Read the model definition and answer for the solid it produces. Units are mm, in the model's axes. Face numbers are marked on the shaded views. A direction names the side the tool comes from. Coordinates: 2 decimals unless noted, no trailing zeros. Loops run counter-clockwise (first coordinate to the right, second up) from the corner with the lowest first, then second, coordinate; pieces in that order, holes last. Notation, with made-up numbers: (76.25, 15.25) - (87.25, 15.25) arc R24 ccw to (87.25, 28.25) - close; hole circle Ø7 at (78.25, 40). An arc over 180 degrees is marked (long way). Use CSV: the item, a comma, the result in double quotes.
Autodesk Inventor part; units mm, degrees
ref_plane "YZ Plane" through (0, 0, 0) normal (1, 0, 0) x (0, 1, 0)
ref_plane "XZ Plane" through (0, 0, 0) normal (0, 1, 0) x (-1, 0, 0)
ref_plane "XY Plane" through (0, 0, 0) normal (0, 0, 1) x (1, 0, 0)
sketch "Skizze7" plane through (0, 0, 0) normal (0, -1, 0) x (1, 0, 0)
  point P0 (-1.8443, 26.478)
sketch "Skizze1" plane through (0, 0, 0) normal (0, 1, 0) x (-1, 0, 0)
  arc A0 (-2.1739, -19.8815) -> (-2.1739, 19.8815) centre (0, 0) ccw
  arc A1 (-47.6304, 14.9111) -> (-47.6304, -14.9111) centre (-46, 0) ccw
  line L0 (-2.1739, 19.8815) -> (-47.6304, 14.9111)
  line L1 (-2.1739, -19.8815) -> (-47.6304, -14.9111)
  line L2 (45.0235, 0) -> (-115.148, 0) construction
  dimension "d0" = 40
  dimension "d1" = 30
  dimension "d2" = 46
extrude "Extrusion1" add sketch "Skizze1" along normal blind 5
shell "Wandung1" thickness 3 removed faces 1 at (17.3261, 5, -4.9704)
sketch "Skizze2" plane through (0, 3, 0) normal (0, 1, 0) x (1, 0, 0)
  circle A0 centre (0, 0) radius 9.5
  circle A1 centre (0, 0) radius 12
  dimension "d6" = 19
  dimension "d7" = 24
extrude "Extrusion2" add sketch "Skizze2" along normal blind 3
sketch "Skizze3" plane through (0, 3, 0) normal (0, 1, 0) x (1, 0, 0)
  arc A0 (47.3043, -11.9289) -> (47.3043, 11.9289) centre (46, 0) ccw
  circle A1 centre (46, 0) radius 9.5
  circle A2 centre (46, 0) radius 12
  point P0 (0, 0)
  point P1 (47.3043, -11.9289)
  dimension "d10" = 19
extrude "Extrusion3" add sketch "Skizze3" along normal blind 3
sketch "Skizze4" plane through (0, 3, 0) normal (0, 1, 0) x (1, 0, 0)
  circle A0 centre (0, 0) radius 9.5
extrude "Extrusion4" cut sketch "Skizze4" against normal blind 2
sketch "Skizze5" plane through (46, 3, 0) normal (0, 1, 0) x (1, 0, 0)
  circle A0 centre (0, 0) radius 9.5
  point P0 (-46, 0)
extrude "Extrusion5" cut sketch "Skizze5" against normal blind 2
sketch "Skizze6" plane through (46, 1, 0) normal (0, 1, 0) x (1, 0, 0)
  point P0 (-46, 0)
  point P1 (0, 0)
  point P2 (0, 0)
hole "Bohrung1" at (46, 1, 0) direction (0, -1, 0) diameter 11 end through all
sketch "Skizze8" plane through (0, 5, 0) normal (0, 1, 0) x (1, 0, 0)
  arc A0 (1.8478, 16.8993) -> (1.8478, -16.8993) centre (0, 0) ccw
  arc A1 (2.1739, 19.8815) -> (2.1739, -19.8815) centre (0, 0) ccw
  line L0 (47.3043, -11.9289) -> (1.8478, -16.8993)
  line L1 (2.1739, -19.8815) -> (47.6304, -14.9111)
  arc A2 (47.6304, -14.9111) -> (47.6304, 14.9111) centre (46, 0) ccw
  circle A3 centre (46, 0) radius 12
  line L2 (1.8478, 16.8993) -> (47.3043, 11.9289)
  line L3 (47.6304, 14.9111) -> (2.1739, 19.8815)
  arc A4 (2.0109, 18.3904) -> (2.0109, -18.3904) centre (0, 0) ccw
  line L4 (2.0109, 18.3904) -> (47.4674, 13.42)
  arc A5 (47.4674, -13.42) -> (47.4674, 13.42) centre (46, 0) ccw
  line L5 (47.4674, -13.42) -> (2.0109, -18.3904)
  line L6 (47.4674, 13.42) -> (46, 0) construction
  line L7 (46, 0) -> (47.4674, -13.42) construction
  line L8 (0, 0) -> (2.0109, -18.3904) construction
  line L9 (0, 0) -> (2.0109, 18.3904) construction
  point P0 (0, -18.5)
  point P1 (56.0514, -9.0122)
  point P2 (59.5, 0)
  point P3 (56.0513, 9.0123)
  point P4 (47.4673, 13.42)
  point P5 (-12.3501, -13.7741)
  point P6 (-18.5, 0)
  point P7 (-12.3501, 13.774)
  point P8 (2.0108, 18.3904)
  point P9 (17.9161, -16.6513)
  point P10 (33.8213, -14.9121)
  point P11 (17.9161, 16.6513)
  point P12 (17.916, 16.6513)
  point P13 (33.8213, 14.9121)
  point P14 (33.8212, 14.9121)
  dimension "d24" = 1.5
  dimension "d26" = 167.52
  dimension "d29" = 167.52
  dimension "d31" = 167.52
  dimension "d34" = 192.48
  dimension "d38" = 16
  dimension "d45" = 16
hole "Bohrung2" at (2.0109, 5, 18.3904) at (-12.3501, 5, 13.7741) at (-18.5, 5, 0) at (-12.3501, 5, -13.774) at (2.0108, 5, -18.3904) at (17.916, 5, -16.6513) at (33.8213, 5, -14.9121) at (47.4673, 5, -13.42) at (56.0513, 5, -9.0123) at (59.5, 5, 0) at (56.0514, 5, 9.0122) at (47.4674, 5, 13.42) at (33.8213, 5, 14.9121) at (17.9161, 5, 16.6513) direction (0, -1, 0) diameter 1 end through all
properties part number "Klapp_Hinten_Abdeckung"
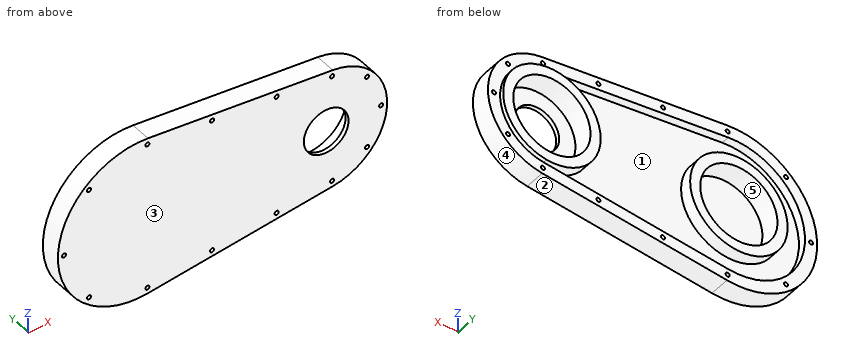
Q1. Find the intervals of material crossed by probe 1 along Z at (x, y) = (0, 4.4); probe 2 along X at (y, z) = (1.45, 0); probe 3 along X at (y, z) = (0.6, 0), in increasing order. Write a range as [from, to].
Reported:
probe 1,"z = [-20, -17], [-12, -9.5], [9.5, 12], [17, 20]"
probe 2,"x = [-20, -19], [-18, -9.5], [9.5, 36.5], [55.5, 59], [60, 61]"
probe 3,"x = [-20, -19], [-18, 40.5], [51.5, 59], [60, 61]"
Q2. For a pull along X with two mould halves and no side action, classify the marked faces 1, 2 and 3 as +X half, -X half, draft (parallel to the pull), parting line (faces both ways), or undercut.
Reported:
face 1,"undercut"
face 2,"+X half"
face 3,"draft"
Q3. Given P1, Ø2, axis at x = 29.5, z = 15, coming from the +Y side; P2, Ø1, axis at y = 3.5, z = -4, coming from the +X side; P3, Ø17, axis at x = 0, z = 0, coming from the +Y side, each flat-ended and moving along its own axis, determine where each tip first touches the part or whether it passes through.
Reported:
P1,"stops at y = 5"
P2,"stops at x = 60.59"
P3,"stops at y = 1"
Q4. A tool of negligible diameter and unlimited length cuts with its end or side. For the marked faces 4 and 5, from which of +Z, -Z, +X, -X, +Y, -Y can it reach the whole face along a straight path? Write none if from no direction.
Reported:
face 4,"+X, +Y, -Y"
face 5,"+Y"
Q5. The part is cut by section C-C on x = -11. Determine the outline of the cut face in (y, z).
Reported:
outline,"(0, -16.7) - (5, -16.7) - (5, -12.96) - (3, -12.96) - (3, -4.8) - (6, -4.8) - (6, 4.8) - (3, 4.8) - (3, 12.96) - (5, 12.96) - (5, 16.7) - (0, 16.7) - close"
Q6. The part is cut by section B-B on z = 4. Determine the outline of the cut face in (x, y), and give its area (3 significant figures).
Reported:
outline,"(-19.6, 0) - (42.23, 0) - (42.23, 1) - (37.38, 1) - (37.38, 6) - (34.69, 6) - (34.69, 3) - (11.31, 3) - (11.31, 6) - (8.62, 6) - (8.62, 1) - (-8.62, 1) - (-8.62, 6) - (-11.31, 6) - (-11.31, 3) - (-16.52, 3) - (-16.52, 5) - (-19.6, 5) - close; (49.77, 0) - (60.46, 0) - (60.46, 5) - (57.31, 5) - (57.31, 6) - (54.62, 6) - (54.62, 1) - (49.77, 1) - close"
area,"208 mm²"
Q7. The part is cut by section A-A on x = 0. Determine the outline of the cut face in (y, z).
Reported:
outline,"(0, -20) - (5, -20) - (5, -17) - (3, -17) - (3, -12) - (6, -12) - (6, -9.5) - (1, -9.5) - (1, 9.5) - (6, 9.5) - (6, 12) - (3, 12) - (3, 17) - (5, 17) - (5, 20) - (0, 20) - close"
